Here's how the part is built. I have some questions about the finished solid (model axes, mm). A direction names the side the tool comes from. Give positions to 0.01 mm unless a question says otherwise; leave off trailing zeros. Order: outer loops, then holes, each group sorted by start corner. A loop starts at its lowest first (then second) coordinate and runs counter-clockwise, first axis right, second up. Notation, with made-up numbers: M -27,-5 L -23,-5 A9 cw -23,10 Z; hole C 2.25,-23 d2. An arc over 180 degrees is marked long. Use one line per item in the form item = value.
from build123d import *

# Parameters (mm, degrees)
F0_W     = 20
F0_H     = 4
F1_DEPTH = 70
F3_DEPTH = 2
F4_R     = 5
F5_DEPTH = 25
F6_R     = 5
F7_DEPTH = 7


with BuildPart() as f1:
    # F0 (on Top) → F1 (new body)
    with BuildSketch(Plane.XY):
        Rectangle(F0_W, F0_H)
    extrude(amount=F1_DEPTH)

    # F2 (on Front) → F3 (join, symmetric)
    with BuildSketch(Plane.XZ):
        with BuildLine():
            Line((-10, 70), (10, 70))
            ThreePointArc((10, 70), (0, 80), (-10, 70))
        make_face()
    extrude(amount=F3_DEPTH, both=True)

    # F4 (on Front) → F5 (cut)
    with BuildSketch(Plane.XZ):
        with Locations((0, 74)):
            Circle(F4_R)
    extrude(amount=F5_DEPTH, mode=Mode.SUBTRACT)

    # F6 (on face) → F7 (join)
    with BuildSketch(Plane.XZ):
        with Locations((0, 74)):
            Circle(F6_R)
    extrude(amount=F7_DEPTH)


solid = f1.part
Q1. I want a section at B-B on y = -6.25. Write out the boundary of the cut face in (x, z), then the cut area to 3 significant figures.
Found:
outline = C 0,74 d10
area = 78.5 mm²
Q2. I want a section at D-D on z = 74. Write out the boundary of the cut face in (x, y).
Found:
outline = M -9.17,-2 L -5,-2 L -5,-7 L 5,-7 L 5,-2 L 9.17,-2 L 9.17,2 L -9.17,2 Z
Q3. On a 3-axis mill with a long thin cutter (end or side, diameter ignored), from which of +Z, -Z, +X, -X, +Y, -Y can I reach the whole of each face in a straight line? I mean faces 1 (the face through (-10, 0, 35)), 2 (the face through (-1.08, -4.46, 69.12)). Say none if no direction works.
Found:
face_1 = +Z, -Z, -X, +Y, -Y
face_2 = -Y
Q4. I'm going to push flat-ended pins straight in: pin 1 Ø1.5 at (x, y) = (-4.5, -6) entering from +Z; pin 2 Ø2 at (x, z) = (7.5, 9.5) entering from -Y; pin 3 Ø1 at (x, y) = (-1.5, -0.5) entering from +Z. Where does each tip first touch, or does it pass through?
Found:
pin_1 = 77.31
pin_2 = -2
pin_3 = 79.95
Q5. I want a section at A-A on x = 0. Write out the boundary of the cut face in (y, z), then the cut area to 3 significant figures.
Found:
outline = M -7,69 L -2,69 L -2,0 L 2,0 L 2,80 L -2,80 L -2,79 L -7,79 Z
area = 370 mm²
Q6. I need wall thicknesses on L1, parallel to Y at x = 1.75, z = 59.5; L2, parallel to Z at x = 0.25, y = -6; L3, parallel to X at y = -3.25, z = 76. Which ranges of each line are inside material? Lowest first, please.
Found:
L1 = -2 to 2
L2 = 69.01 to 78.99
L3 = -4.58 to 4.58
Q7. I want a section at C-C on z = 59.5. Write out the boundary of the cut face in (x, y), then the cut area to 3 significant figures.
Found:
outline = M -10,-2 L 10,-2 L 10,2 L -10,2 Z
area = 80.0 mm²
